Autodesk Inventor part; units mm, degrees
ref_plane "Work Plane2" through (-123, 0, 0) normal (1, 0, 0) x (0, 1, 0)
ref_plane "XZ Plane" through (0, 0, 0) normal (0, 1, 0) x (-1, 0, 0)
ref_plane "XY Plane" through (0, 0, 0) normal (0, 0, 1) x (1, 0, 0)
sketch "Sketch1" plane through (0, 0, 0) normal (1, 0, 0) x (0, 1, 0)
  circle A0 centre (0, 0) radius 12.5
  circle A1 centre (0, 0) radius 10
  dimension "d0" = 25
  dimension "d1" = 20
extrude "Extrusion1" add sketch "Sketch1" against normal blind 130 contours A0 | A1
extrude "Extrusion2" cut sketch "Sketch1" against normal blind 100
ref_plane "Work Plane2" through (-123, 0, 0) normal (1, 0, 0) x (0, 1, 0)
sketch "Sketch4" plane through (-123, 0, 0) normal (1, 0, 0) x (0, 1, 0)
  circle A0 centre (0, 0) radius 7.5
  circle A1 centre (0, 0) radius 9.5
  dimension "d11" = 15
  dimension "d20" = 19
extrude "Extrusion4" cut sketch "Sketch4" along normal blind 6
sketch "Sketch5" plane through (0, 0, 0) normal (1, 0, 0) x (0, 0, -1)
  line L0 (-7, 3) -> (-9.5394, 3)
  line L1 (-7, 3) -> (-7, -3)
  line L2 (-7, -3) -> (-9.5394, -3)
  circle A0 centre (0, 0) radius 10
  arc A1 (-9.5394, 3) -> (-9.5394, -3) centre (0, 0) ccw
  point P0 (-7, 0)
  dimension "d14" = 7
  dimension "d15" = 6
  dimension "d16" = 3
extrude "Extrusion5" cut sketch "Sketch5" against normal blind 20 contours L1 L2 A0 L0 picked at (-7.9828, -0.338)
sketch "Sketch6" plane through (-130, 0, 0) normal (-1, 0, 0) x (0, 0, 1)
  circle A0 centre (0, 0) radius 12.5
  circle A1 centre (0, 0) radius 9.5
  dimension "d21" = 19
extrude "Extrusion6" cut sketch "Sketch6" against normal blind 20
properties part number "shaft" material "Stainless Steel, 440C"
Geometry: final body of the model. Coordinates: model frame, mm. A direction names the side the tool comes from. Round coordinates to 2 decimals unless told otherwise and drop trailing zeros. Loops run counter-clockwise (first coordinate to the right, second up) from the corner with the lowest first, then second, coordinate; pieces in that order, holes last. Notation, with made-up numbers: (23, 33) -> (37, 33) arc R7 ccw to (37, 40) -> close; hole circle Ø7 at (24, 4). An arc over 180 degrees is marked (long way). Use one line per item in the form item = value. Start each with the question number.
1) First-contact query: P1, Ø6, axis at x = -73, y = 3.5, coming from the +Z side; P2, Ø2, axis at x = -75.5, z = 9, coming from the +Y side; P3, Ø6, axis at x = -90.5, z = -2, coming from the +Y side. Flat tips, straight axial feed; report the tip coordinate or a pass-through.
2) Section B-B on y = 0. Output: boundary loops of the cut face in (x, z).
3) Section A-A on z = 0. Output: boundary loops of the cut face in (x, y), then the cut area to 3 significant figures.
4) Line query: L1, parallel to X at y = 4, z = -7; L2, parallel to X at y = 2.25, z = 8; L3, parallel to X at y = 4.5, z = 10. Output: solid intervals per line, ascending.
5) Access query for faces 4 (the cylindrical face through (-120.042, -7.493, -0.33)), 5 (the cylindrical face through (-49.3, -2.17, -9.76)), 6 (the cylindrical face through (-113.55, -8.43, 4.38)), 7 (the flat face through (-10, -3, 8)). Directions: +Z, -Z, +X, -X, +Y, -Y. A direction counts if a zero-diameter tool reaches every point of the face in a straight line with its end or side. Return the directions, or none.
6) Draft query along X for faces 1 (the flat face through (-110, 9.3, 2.7)), 2 (the flat face through (-123, 1, 8)), 3 (the cylindrical face through (-126.55, -8.43, 4.38)). Return one class per face: released by +X, released by -X, zero draft, split by the parting line, or undercut.
7) Section D-D on x = -113.5. Output: boundary loops of the cut face in (y, z).
8) Section C-C on x = -12. Output: boundary loops of the cut face in (y, z).
Response:
q1.P1 = 9.99
q1.P2 = 6
q1.P3 = 10
q2.outline = (-130, -9.5) -> (-123, -9.5) -> (-123, -7.5) -> (-117, -7.5) -> (-117, -9.5) -> (-110, -9.5) -> (-110, -12.5) -> (-100, -12.5) -> (-100, -10) -> (0, -10) -> (0, 7) -> (-20, 7) -> (-20, 10) -> (-100, 10) -> (-100, 12.5) -> (-110, 12.5) -> (-110, 9.5) -> (-117, 9.5) -> (-117, 7.5) -> (-123, 7.5) -> (-123, 9.5) -> (-130, 9.5) -> close
q3.outline = (-130, -9.5) -> (-123, -9.5) -> (-123, -7.5) -> (-117, -7.5) -> (-117, -9.5) -> (-110, -9.5) -> (-110, -12.5) -> (-100, -12.5) -> (-100, -10) -> (0, -10) -> (0, 10) -> (-100, 10) -> (-100, 12.5) -> (-110, 12.5) -> (-110, 9.5) -> (-117, 9.5) -> (-117, 7.5) -> (-123, 7.5) -> (-123, 9.5) -> (-130, 9.5) -> close
q3.area = 2,610 mm^2
q4.L1 = -130 to -123, -117 to 0
q4.L2 = -130 to -123, -117 to -20
q4.L3 = -110 to -100
q5.face_4 = none
q5.face_5 = +X
q5.face_6 = -X
q5.face_7 = +Z, +X
q6.face_1 = released by -X
q6.face_2 = undercut
q6.face_3 = zero draft
q7.outline = circle Ø19 at (0, 0)
q8.outline = (-3, 7) -> (-3, 9.54) arc R10 ccw (long way) to (3, 9.54) -> (3, 7) -> close
